Solid Edge part; units mm, degrees
sketch "Sketch1" plane through (0, 0, 0) normal (0, -1, 0) x (1, 0, 0)
  line L0 (-25, -20) -> (25, -20)
  line L1 (25, -20) -> (25, 20)
  line L2 (25, 20) -> (-25, 20)
  line L3 (-25, 20) -> (-25, -20)
  dimension "D1" = 25
  dimension "D2" = 25
extrude "Protrusion1" add sketch "Sketch1" along normal mid plane 40
sketch "Sketch2" plane through (0, -20, 0) normal (0, -1, 0) x (1, 0, 0)
  line L0 (0, 20) -> (-13.8266, 20)
  line L1 (-13.8266, 20) -> (0, 0)
  line L2 (0, 0) -> (12.0573, 20)
  line L3 (12.0573, 20) -> (0, 20)
extrude "ExtrudedCutout_1" cut sketch "Sketch2" against normal blind 20
For this review, take the finished solid that the model builds, in its own axes (mm). A direction names the side the tool comes from. Give positions to 0.01 mm unless a question says otherwise; leave off trailing zeros. Order: outer loops, then holes, each group sorted by start corner. A loop starts at its lowest first (then second) coordinate and runs counter-clockwise, first axis right, second up. Notation, with made-up numbers: (11.5, 46) -> (30.5, 46) arc R20 cw to (30.5, 59) -> close; hole circle Ø5 at (86.25, -19). An arc over 180 degrees is marked (long way). Write item = value, one per line.
1) We need section A-A, the plane y = -10. Give the boundary of the cut face in (x, z).
Findings:
outline = (-25, -20) -> (25, -20) -> (25, 20) -> (12.06, 20) -> (0, 0) -> (-13.83, 20) -> (-25, 20) -> close
2) For faces 4 (the face through (0.4, -20, 0.3)), 5 (the face through (5.944, -10.14, 9.86)), list the 3-axis set-ups (+Z, -Z, +X, -X, +Y, -Y) from which the entire face can be reached by the end or side of a thin tool; tool diameter is ignored.
Findings:
face_4 = +Z, -Z, +X, -X, -Y
face_5 = +Z, -Y
3) Insertion check: pin 1 (2 mm diameter, centred on x = 4, z = 12.5, fed in from -Y). The pin has a flat end and moves straight along its axis. Give the tip position at first contact, or say it passes through.
Findings:
pin_1 = 0
4) To check wall thickness, follow L1, parallel to X at y = -14, z = 15.5; L2, parallel to X at y = -12.5, z = 14.5; L3, parallel to Y at x = 0.5, z = 7. State the ranges of each line that lie inside material, in increasing order. Write a range as from..to.
Findings:
L1 = -25..-10.72, 9.34..25
L2 = -25..-10.02, 8.74..25
L3 = 0..20
5) Draft analysis for pull direction X (two halves, no side actions). For faces 1 (the face through (0, 20, 0)), 2 (the face through (-7.01, -10.14, 10.14)), 3 (the face through (25, 0, 0)), state which applies: pulls with the +X half, pulls with the -X half, needs draft (parallel to the pull), parting line crosses it, or undercut.
Findings:
face_1 = needs draft
face_2 = undercut
face_3 = pulls with the +X half
6) We need section D-D, the plane z = 2. Give the boundary of the cut face in (x, y), and give its area (3 significant figures).
Findings:
outline = (-25, -20) -> (-1.38, -20) -> (-1.38, 0) -> (1.21, 0) -> (1.21, -20) -> (25, -20) -> (25, 20) -> (-25, 20) -> close
area = 1,950 mm^2
7) We need section C-C, the plane x = -5. Give the boundary of the cut face in (y, z).
Findings:
outline = (-20, -20) -> (20, -20) -> (20, 20) -> (0, 20) -> (0, 7.23) -> (-20, 7.23) -> close
8) We need section B-B, the plane z = 10. Give the boundary of the cut face in (x, y).
Findings:
outline = (-25, -20) -> (-6.91, -20) -> (-6.91, 0) -> (6.03, 0) -> (6.03, -20) -> (25, -20) -> (25, 20) -> (-25, 20) -> close
